Part print with two shaded views. Sizes in mm from the minimum x, y, z corner. A direction names the side the tool comes from. Give positions to 0.01 mm unless a question says otherwise; leave off trailing zeros. Write each loop counter-clockwise with the first axis right and the second up, starting at its lowest first coordinate (ties: lowest second). Pieces come first, ordered by that corner, then holes. Notation, with made-up numbers: (58, 7) - (89, 7) arc R17 cw to (89, 15) - close; hole circle Ø9 at (-34.75, 22.5). An arc over 180 degrees is marked (long way). One line per item, written item: value. Start each with the question number.
(1) Cut at D-D, the plane x = 7. List the corners of the cut face in (y, z).
(2) 3-axis set-ups, long thin cutter, end or side, ignore diameter. For the marked faces 1 and 2: which of +Z, -Z, +X, -X, +Y, -Y reach the whole face in a straight line?
(3) Cut at B-B, the plane z = 34.93. List the corners of the cut face in (x, y), and give its area (4 significant figures).
(4) Drop a flat-ended pin along its axis: P1, Ø6, axis at x = 41.5, y = 113, coming from the -Z side. Give the stop position or say it passes through.
(5) Cut at C-C, the plane y = 155. List the corners of the cut face in (x, z), and give its area (3 significant figures).
(6) Probe L1, parallel to Y at x = 48, z = 34.93; L2, parallel to Z at x = 21.5, y = 69; L3, parallel to X at y = 67, z = 27. List the from-to ranges inside material, lowest first.
(7) Cut at A-A, the plane y = 127. List the corners of the cut face in (x, z), and give its area (3 significant figures).
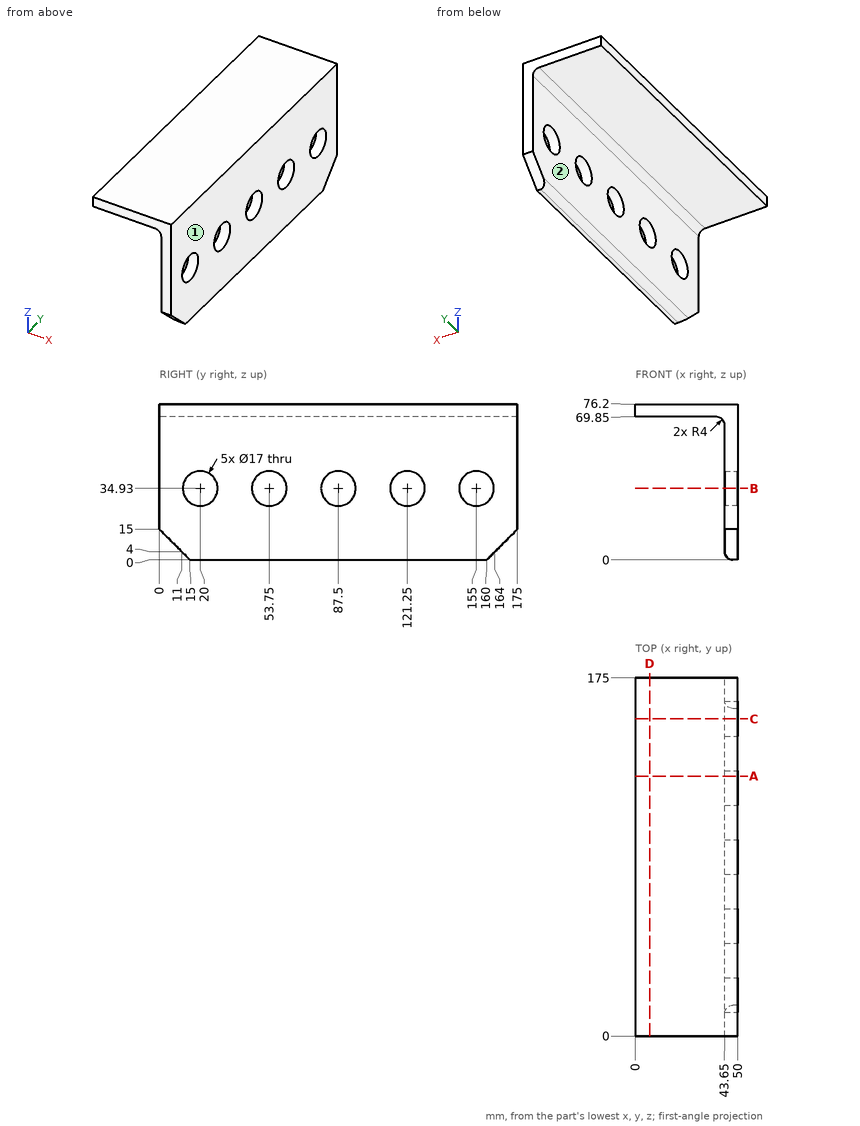
Answers follow:
1. outline: (0, 69.85) - (175, 69.85) - (175, 76.2) - (0, 76.2) - close
2. face 1: +Z, -Z, +X, +Y, -Y
2. face 2: -Z, -X, +Y, -Y
3. outline: (43.65, 0) - (50, 0) - (50, 11.5) - (43.65, 11.5) - close; (43.65, 28.5) - (50, 28.5) - (50, 45.25) - (43.65, 45.25) - close; (43.65, 62.25) - (50, 62.25) - (50, 79) - (43.65, 79) - close; (43.65, 96) - (50, 96) - (50, 112.75) - (43.65, 112.75) - close; (43.65, 129.75) - (50, 129.75) - (50, 146.5) - (43.65, 146.5) - close; (43.65, 163.5) - (50, 163.5) - (50, 175) - (43.65, 175) - close
3. area: 571.5 mm²
4. P1: stops at z = 1.53
5. outline: (0, 69.85) - (39.65, 69.85) arc R4 cw to (43.65, 65.85) - (43.65, 43.43) - (50, 43.43) - (50, 76.2) - (0, 76.2) - close; (43.65, 4) arc R4 ccw to (47.65, 0) - (50, 0) - (50, 26.43) - (43.65, 26.43) - close
5. area: 653 mm²
6. L1: y = 0 to 11.5, 28.5 to 45.25, 62.25 to 79, 96 to 112.75, 129.75 to 146.5, 163.5 to 175
6. L2: z = 69.85 to 76.2
6. L3: x = 43.65 to 50
7. outline: (0, 69.85) - (39.65, 69.85) arc R4 cw to (43.65, 65.85) - (43.65, 41.19) - (50, 41.19) - (50, 76.2) - (0, 76.2) - close; (43.65, 4) arc R4 ccw to (47.65, 0) - (50, 0) - (50, 28.67) - (43.65, 28.67) - close
7. area: 682 mm²
